For this review, use the dimensioned drawing (mm, ordinates from the lowest corner) and the shaded views. Give positions to 0.01 mm unless a question says otherwise; leave off trailing zeros. Order: outer loops, then holes, each group sorted by start corner. A loop starts at its lowest first (then second) coordinate and runs counter-clockwise, first axis right, second up.
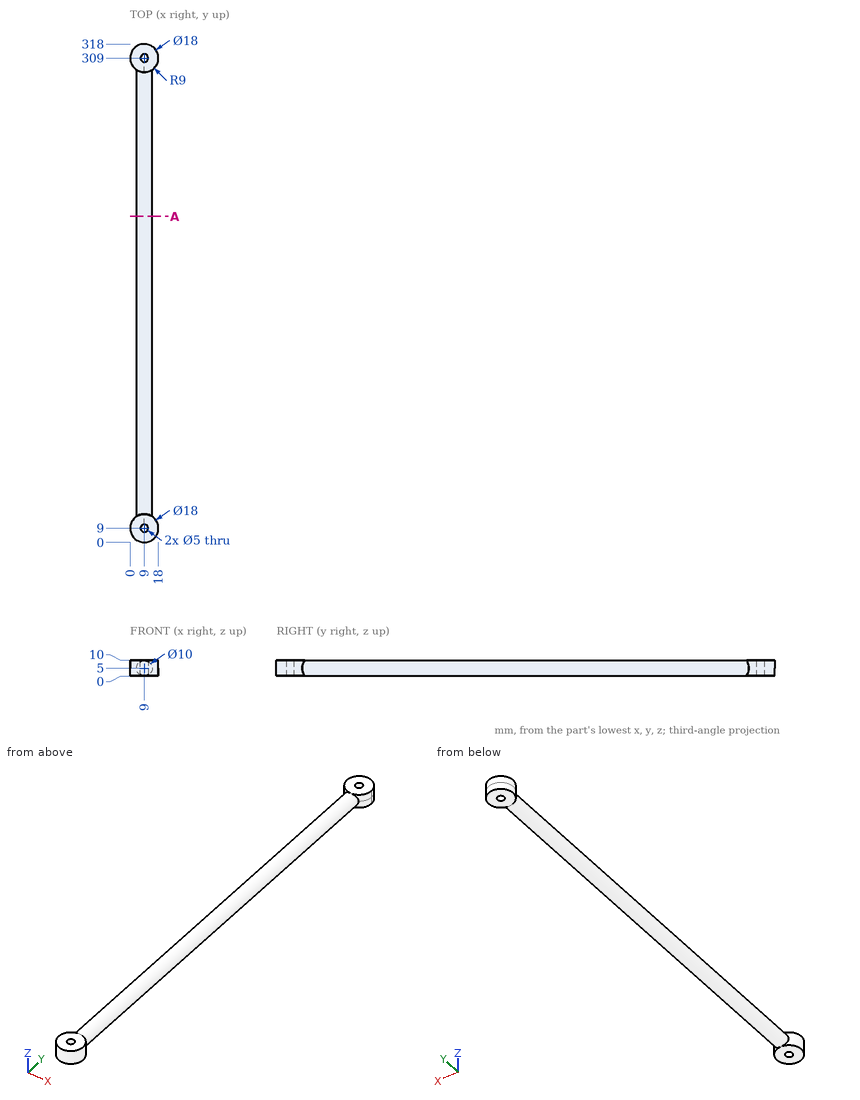
1. For line 1 along Y through (x, z) = (7.25, 1); line 2 along Y through (x, z) = (2.75, 8.25); line 3 along Y through (x, z) = (14, 9.25), list the stretches that pass through material, from the lowest coordinate up.
Recorded:
line 1: y = 0.17 to 7.21, 10.79 to 307.21, 310.79 to 317.83
line 2: y = 2.52 to 15.48, 302.52 to 315.48
line 3: y = 1.52 to 16.48, 301.52 to 316.48
2. For pin 1 (5 mm diameter, centred on x = 13, z = 7, fed in from +Y); pin 2 (2 mm diameter, centred on x = 7.5, y = 112, fed in from +Z); pin 3 (8 mm diameter, centred on x = 3.5, y = 170, fed in from -Z), all flat-tipped, find the tip position at first contact; note any pin that passes through.
Recorded:
pin 1: stops at y = 317.87
pin 2: stops at z = 9.97
pin 3: stops at z = 0.23
3. Take a section at A-A (y = 208). State the section outline as (x, z) points, then the cut area to 3 significant figures.
Recorded:
outline: circle Ø10 at (9, 5)
area: 78.5 mm2
